Input: part model. Units: mm. Frame: model coordinates. Face numbers are marked on the shaded views. A direction names the side the tool comes from. Coordinates: 2 decimals unless noted, no trailing zeros. Loops run counter-clockwise (first coordinate to the right, second up) from the corner with the lowest first, then second, coordinate; pieces in that order, holes last. Notation, with made-up numbers: (54.5, 10.25) -> (105.5, 10.25) arc R25 ccw to (105.5, 28.25) -> close; hole circle Ø6 at (30, 8). An arc over 180 degrees is marked (long way). Answer as a JSON object with one key per item and string values.
Autodesk Inventor part; units mm, degrees
ref_plane "YZ Plane" through (0, 0, 0) normal (1, 0, 0) x (0, 1, 0)
ref_plane "XZ Plane" through (0, 0, 0) normal (0, 1, 0) x (-1, 0, 0)
ref_plane "XY Plane" through (0, 0, 0) normal (0, 0, 1) x (1, 0, 0)
sketch "Sketch1" plane through (0, 0, 0) normal (0, 1, 0) x (-1, 0, 0)
  line L0 (0, 0) -> (50.292, 0)
  line L1 (50.292, 0) -> (50.292, -62.992)
  line L2 (50.292, -62.992) -> (0, -62.992)
  line L3 (0, -62.992) -> (0, 0)
  line L4 (50.292, -22.225) -> (57.912, -22.225)
  line L5 (57.912, -22.225) -> (57.912, -41.2242)
  line L6 (57.912, -41.2242) -> (50.292, -41.2242)
  line L7 (50.292, -41.2242) -> (50.292, -22.225)
  dimension "d0" = 50.292
  dimension "d1" = 62.992
  dimension "d2" = 7.62
  dimension "d3" = 18.9992
  dimension "d4" = 22.225
extrude "Extrusion1" add sketch "Sketch1" against normal blind 1.27 contours L0 L1 L2 L3
extrude "Extrusion2" add sketch "Sketch1" against normal blind 4.572 contours L4 L5 L6 L1
sketch "Sketch2" plane through (-57.912, 0, -22.225) normal (0, 0, 1) x (1, 0, 0)
  line L0 (7.62, 0) -> (0, 0)
  line L1 (1.27, 0) -> (6.35, 0)
  line L2 (6.35, 0) -> (6.35, -1.27)
  line L3 (3.81, -3.81) -> (3.81, -3.81)
  line L4 (1.27, -1.27) -> (1.27, 0)
  line L5 (0, 0) -> (0, -4.572)
  arc A0 (1.27, -1.27) -> (3.81, -3.81) centre (3.81, -1.27) ccw
  arc A1 (3.81, -3.81) -> (6.35, -1.27) centre (3.81, -1.27) ccw
  point P0 (57.912, 0)
  point P1 (6.35, -3.81)
  point P2 (1.27, -3.81)
  point P3 (3.81, -3.81)
  point P4 (6.35, 0)
  dimension "d9" = 5.08
  dimension "d10" = 3.81
  dimension "d11" = 1.27
  dimension "d12" = 2.54
  dimension "d13" = 2.54
extrude "Extrusion3" cut sketch "Sketch2" against normal through all
fillet "Fillet1" radius 3.175 2 edges at (-50.292, -4.572, -31.7246) (-57.912, -4.572, -31.7246)
properties part number "Battery Cover" material "PC/ABS Plastic"
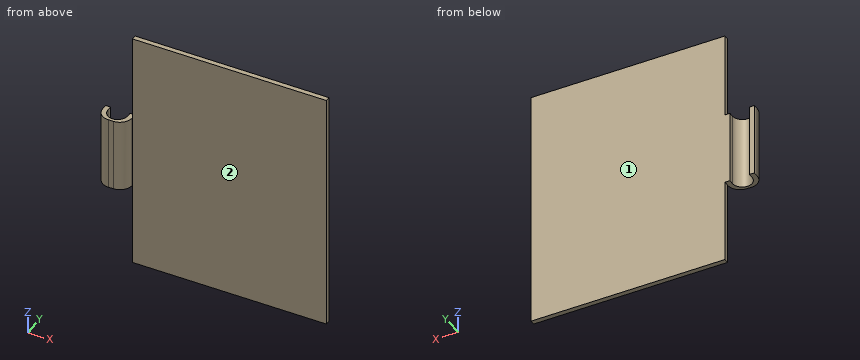
1. Section query A-A (z = -29.5). Return loops of the section in (x, y) (3 decimals), plus the area to 3 significant figures.
Reply:
{"outline": "(-57.912, -1.397) arc R3.175 ccw to (-54.737, -4.572) -> (-53.467, -4.572) arc R3.175 ccw to (-50.292, -1.397) -> (-50.292, -1.27) -> (0, -1.27) -> (0, 0) -> (-51.562, 0) -> (-51.562, -1.27) arc R2.54 cw to (-56.642, -1.27) -> (-56.642, 0) -> (-57.912, 0) -> close", "area": "77.8 mm2"}
2. Section query B-B (y = -2.2). Return loops of the section in (x, z) (3 decimals).
Reply:
{"outline": "(-57.809, -41.224) -> (-56.466, -41.224) -> (-56.466, -22.225) -> (-57.809, -22.225) -> close; (-51.738, -41.224) -> (-50.395, -41.224) -> (-50.395, -22.225) -> (-51.738, -22.225) -> close"}
3. Access query for the marked faces 1 and 2. Directions: +Z, -Z, +X, -X, +Y, -Y. A direction counts if a zero-diameter tool reaches every point of the face in a straight line with its end or side. Return the directions, or none.
Reply:
{"face 1": "+Z, -Z, +X, -X, +Y", "face 2": "+Z, -Z, +X, -Y"}
4. Section query C-C (x = -6.5). Return loops of the section in (y, z).
Reply:
{"outline": "(-1.27, -62.99) -> (0, -62.99) -> (0, 0) -> (-1.27, 0) -> close"}
5. Section query D-D (z = -16.5). Return loops of the section in (x, y), plus the area to 3 significant figures.
Reply:
{"outline": "(-50.29, -1.27) -> (0, -1.27) -> (0, 0) -> (-50.29, 0) -> close", "area": "63.9 mm2"}
6. Pin query (flat end, axial travel): P1, Ø1, axis at x = -11, y = -2.5, coming from the +Z side; P2, Ø1.5, axis at y = -1.5, z = -46.5, coming from the -X side; P3, Ø25, axis at x = -22, z = -30, coming from the -Y side. Return the tip coordinate at first contact, or that it passes through.
Reply:
{"P1": "passes through", "P2": "stops at x = -50.29", "P3": "stops at y = -1.27"}
7. Line query: line 1 along Y through (x, z) = (-8, -36); line 2 along X through (y, z) = (-0.55, -4.5); line 3 along X through (y, z) = (-1.5, -37.5). Output: solid intervals per line, ascending.
Reply:
{"line 1": "y = -1.27 to 0", "line 2": "x = -50.29 to 0", "line 3": "x = -57.91 to -56.63, -51.57 to -50.29"}
